Model file for the job. Use its own axes, mm. A direction names the side the tool comes from. Coordinates: 2 decimals unless noted, no trailing zeros. Write each loop counter-clockwise with the first axis right and the second up, starting at its lowest first coordinate (ties: lowest second). Pieces come first, ordered by that corner, then holes. Notation, with made-up numbers: M 74,59.5 L 81,59.5 A24 cw 81,69.5 Z; hole C -35,47.5 d1. An arc over 180 degrees is marked long. Put each result on its own line as item: value. Start each with the question number.
Q1. Cut at B-B (x = -25). Write the cut outline in (y, z).
Q2. Drill centre lines: line 1 along Y through (x, z) = (-95, 177); line 2 along X through (y, z) = (-162, 250); line 3 along Z through (x, y) = (-71, 191). Where is each one in solid material? Low to high.
Q3. Which spindle directions (+Z, -Z, +X, -X, +Y, -Y) get a long thin tool onto all of the face, cutting with end or side? Do faces 5 (the cylindrical face through (-194.297, 218.986, 161.96)), 6 (the cylindrical face through (192.587, -217.867, 161.96)). Say none if no direction does.
Q4. Pull direction X, two halves, no side cores. Call faces 1 (the flat face through (-3, 3, 0)), 2 (the cylindrical face through (193.986, -219.297, 161.96)), 3 (the flat face through (-200, -3, 158)), 4 (the flat face through (-3, 223, 158)): pulls with the +X half, pulls with the -X half, needs draft (parallel to the pull), parting line crosses it, or undercut.
Q5. Cut at A-A (z = 120.5). Write the cut outline in (x, y), then the cut area to 3 significant figures.
Q6. Cut at C-C (y = -52.5). Write the cut outline in (x, z).
```python
from build123d import *

# Parameters (mm, degrees)
SKIZZE1_W                       = 400
SKIZZE1_H                       = 450
AUFSATZ_LINEAR_AUSTRAGEN1_DEPTH = 300
VERRUNDUNG2_R                   = 20
WANDUNG1_T                      = -2


with BuildPart() as part:
    # Skizze1 → Aufsatz-Linear austragen1 (new body)
    with BuildSketch(Plane.XY):
        Rectangle(SKIZZE1_W, SKIZZE1_H)
    extrude(amount=AUFSATZ_LINEAR_AUSTRAGEN1_DEPTH)

    # Verrundung2
    verrundung2_edges = [part.edges().sort_by_distance(p)[0] for p in [
        (0, -225, 0),
        (-200, 0, 0),
        (0, 225, 0),
        (200, 0, 0),
        (200, -225, 150),
        (-200, -225, 150),
        (-200, 225, 150),
        (200, 225, 150),
    ]]
    fillet(verrundung2_edges, radius=VERRUNDUNG2_R)

    # Wandung1
    wandung1_openings = [part.faces().sort_by_distance(p)[0] for p in [
        (0, 0, 300),
    ]]
    offset(amount=WANDUNG1_T, openings=wandung1_openings, kind=Kind.INTERSECTION)


solid = part.part
```
Computed values:
1. outline: M -225,20 A20 ccw -205,0 L 205,0 A20 ccw 225,20 L 225,300 L 223,300 L 223,20 A18 cw 205,2 L -205,2 A18 cw -223,20 L -223,300 L -225,300 Z
2. line 1: -225 to -223, 223 to 225
2. line 2: -200 to -198, 198 to 200
2. line 3: 0 to 2
3. face 5: +Z, -Z, -X, +Y
3. face 6: +Z
4. face 1: needs draft
4. face 2: pulls with the +X half
4. face 3: pulls with the -X half
4. face 4: undercut
5. outline: M -200,-205 A20 ccw -180,-225 L 180,-225 A20 ccw 200,-205 L 200,205 A20 ccw 180,225 L -180,225 A20 ccw -200,205 Z; hole M -198,-205 A18 ccw -180,-223 L 180,-223 A18 ccw 198,-205 L 198,205 A18 ccw 180,223 L -180,223 A18 ccw -198,205 Z
5. area: 3,320 mm2
6. outline: M -200,20 A20 ccw -180,0 L 180,0 A20 ccw 200,20 L 200,300 L 198,300 L 198,20 A18 cw 180,2 L -180,2 A18 cw -198,20 L -198,300 L -200,300 Z
